The model under review builds one solid part; all positions refer to its coordinate system, in mm. A direction names the side the tool comes from. Give positions to 0.01 mm unless a question says otherwise; leave off trailing zeros. Order: outer loops, then holes, each group sorted by start corner. A loop starts at its lowest first (then second) coordinate and runs counter-clockwise, first axis right, second up. Notation, with made-up numbers: (37.25, 7.5) - (71.25, 7.5) arc R21 ccw to (71.25, 31.5) - close; hole circle Ø4 at (20, 21). An arc over 180 degrees is marked (long way). Use a Markdown table: item, result. Add a question column.
```python
from build123d import *

# Parameters (mm, degrees)
F1_DEPTH = 4
F2_W     = 34.5
F2_H     = 45.5
F3_DEPTH = 1
F4_R     = 1.75
F5_DEPTH = 25


with BuildPart() as f1:
    # F0 (on Top) → F1 (new body)
    with BuildSketch(Plane.XY):
        Polygon((26, 5), (26, 29), (-26, 29), (-26, 5), (-36, 5), (-36, -5), (-26, -5), (-26, -29), (26, -29), (26, -5), (36, -5), (36, 5), align=None)
    extrude(amount=F1_DEPTH)

    # F2 (on Top) → F3 (cut)
    with BuildSketch(Plane.XY):
        with Locations((0, 5.032895)):
            Rectangle(F2_W, F2_H)
    extrude(amount=F3_DEPTH, mode=Mode.SUBTRACT)

    # F4 (on Top) → F5 (cut)
    with BuildSketch(Plane.XY):
        with Locations((-18.500006, -21.499975)):
            Circle(F4_R)
        with Locations((18.49998, -21.499971)):
            Circle(F4_R)
        with Locations((-20.999989, 21.499986)):
            Circle(F4_R)
        with Locations((21.000014, 21.499973)):
            Circle(F4_R)
        with Locations((-30.999894, 0)):
            Circle(F4_R)
        with Locations((30.99998, 0)):
            Circle(F4_R)
    extrude(amount=F5_DEPTH, mode=Mode.SUBTRACT)


solid = f1.part
```
Q1. Clearance check with flat-ended pins moving along their axes: P1, Ø1.2, axis at x = -32, z = 3, coming from the +Y side; P2, Ø2, axis at y = 14.5, z = 3, coming from the +X side; P3, Ø2, axis at x = -29.5, z = 2.5, coming from the -Y side; P4, Ø2, axis at x = 21, y = 21.5, coming from the -Z side. State where each tip first meets the part, or that it passes through.
Q2. We need section D-D (y = 12.5). Write out the cut boundary in (x, z).
Q3. We need section A-A (y = 0). Write out the cut boundary in (x, z).
Q4. Machinability: for faces 5 (the flat face through (31, 5, 2)), 6 (the flat face through (-26, 17, 2)), 7 (the flat face through (-31, -5, 2)), which of the approach directions +Z, -Z, +X, -X, +Y, -Y give a long, thin tool a straight path to every point of the face, cutting with its end or side? Answer none if there is none.
Q5. We need section B-B (x = 14). Write out the cut boundary in (y, z), plus the area to 4 significant figures.
Q6. Draft analysis for pull direction Y (two halves, no side actions). For faces 1 (the cylindrical face through (-22.29, 22.68, 1.97)), 2 (the flat face through (31, -5, 2)), 3 (the cylindrical face through (20.772, 23.235, 1.972)), 4 (the flat face through (-36, 0, 2)), state which applies: pulls with the +Y half, pulls with the -Y half, needs draft (parallel to the pull), parting line crosses it, or undercut.
Q7. We need section C-C (z = 3). Write out the cut boundary in (x, y), plus the area to 3 significant figures.
Q8. Wall thickness on probe 1 along X at (y, z) = (0, 1.9); probe 2 along X at (y, z) = (-21, 3.85); probe 3 along Z at (x, y) = (-6, 19.5): over which ranges is each line inside the solid? List them lowest first.
Here are the results:
| question | item | result |
|---|---|---|
| 1 | P1 | y = 5 |
| 1 | P2 | x = 26 |
| 1 | P3 | y = -5 |
| 1 | P4 | through |
| 2 | outline | (-26, 0) - (-17.25, 0) - (-17.25, 1) - (17.25, 1) - (17.25, 0) - (26, 0) - (26, 4) - (-26, 4) - close |
| 3 | outline | (-36, 0) - (-32.75, 0) - (-32.75, 4) - (-36, 4) - close; (-29.25, 0) - (-17.25, 0) - (-17.25, 1) - (17.25, 1) - (17.25, 0) - (29.25, 0) - (29.25, 4) - (-29.25, 4) - close; (32.75, 0) - (36, 0) - (36, 4) - (32.75, 4) - close |
| 4 | face 5 | +Z, -Z, +X, +Y |
| 4 | face 6 | +Z, -Z, -X, +Y |
| 4 | face 7 | +Z, -Z, -X, -Y |
| 5 | outline | (-29, 0) - (-17.72, 0) - (-17.72, 1) - (27.78, 1) - (27.78, 0) - (29, 0) - (29, 4) - (-29, 4) - close |
| 5 | area | 186.5 mm2 |
| 6 | face 1 | undercut |
| 6 | face 2 | pulls with the -Y half |
| 6 | face 3 | undercut |
| 6 | face 4 | needs draft |
| 7 | outline | (-36, -5) - (-26, -5) - (-26, -29) - (26, -29) - (26, -5) - (36, -5) - (36, 5) - (26, 5) - (26, 29) - (-26, 29) - (-26, 5) - (-36, 5) - close; hole circle Ø3.5 at (-31, 0); hole circle Ø3.5 at (-21, 21.5); hole circle Ø3.5 at (-18.5, -21.5); hole circle Ø3.5 at (18.5, -21.5); hole circle Ø3.5 at (21, 21.5); hole circle Ø3.5 at (31, 0) |
| 7 | area | 3,160 mm2 |
| 8 | probe 1 | -36 to -32.75, -29.25 to 29.25, 32.75 to 36 |
| 8 | probe 2 | -26 to -20.18, -16.82 to 16.82, 20.18 to 26 |
| 8 | probe 3 | 1 to 4 |
